from build123d import *

# Parameters (mm, degrees)
SKETCH1_W          = 201.20864
SKETCH1_H          = 290.83
BASE_FLANGE1_DEPTH = 3.175
EDGE_FLANGE1_DEPTH = 93.921520056


# Sheet-metal steps are written as plain solids
with BuildPart() as part:
    # Sketch1 → Base-Flange1 (new body)
    with BuildSketch(Plane(origin=(0, 0, 0), x_dir=(1, 0, 0), z_dir=(0, 1, 0))):
        with Locations((100.60432, 145.415)):
            Rectangle(SKETCH1_W, SKETCH1_H)
    extrude(amount=-BASE_FLANGE1_DEPTH)

    # Edge-Flange1 section (across the edge) → Edge-Flange1 (add)
    with BuildSketch(Plane(origin=(93.921520056, 0, -294.005), x_dir=(0, 0, 1), z_dir=(-1, 0, 0))):
        with BuildLine():
            Line((-3.175, 3.175), (-3.175, 34.925))
            Line((-3.175, 34.925), (0, 34.925))
            Line((0, 34.925), (0, 3.175))
            ThreePointArc((0, 3.175), (0.92993597, 0.92993597), (3.175, 0))
            Line((3.175, 0), (3.175, -3.175))
            ThreePointArc((3.175, -3.175), (-1.315128061, -1.315128061), (-3.175, 3.175))
        make_face()
    extrude(amount=EDGE_FLANGE1_DEPTH)


solid = part.part
Model file for the job. Use its own axes, mm. A direction names the side the tool comes from. Round coordinates to 2 decimals unless told otherwise and drop trailing zeros. Order: outer loops, then holes, each group sorted by start corner. A loop starts at its lowest first (then second) coordinate and runs counter-clockwise, first axis right, second up.
(1) Band-saw the part on A-A (x = 54). List the corners of the cut face in (y, z) (3 decimals).
(2) Band-saw the part on B-B (y = 24). List the corners of the cut face in (x, z) (3 decimals).
(3) Band-saw the part on C-C (z = -226). List the corners of the cut face in (x, y) (3 decimals), then the cut area to 3 significant figures.
(4) Drill centre lines: line 1 (Z direction, x = 50, y = 30) (3 decimals); line 2 (Y direction, x = 50, z = -212) (3 decimals). Where is each one in solid material? Low to high.
(5) Pin check, flat tips, straight feed: pin 1 (1.9 mm diameter, centred on y = 18.5, z = -295.5, fed in from +X); pin 2 (16 mm diameter, centred on x = 51, y = 24, fed in from +Z) (3 decimals); pin 3 (1.6 mm diameter, centred on x = 155, y = -2.5, fed in from -Z). Stop position of each tip, or through.
(6) 3-axis set-ups, long thin cutter, end or side, ignore diameter. For faces 1 (the face through (48, 19, -294.005)), 2 (the face through (93.922, 16, -295)), 3 (the face through (0, -1, -148)): which of +Z, -Z, +X, -X, +Y, -Y reach the whole face in a straight line?
Verdict:
1. outline: (-3.175, -290.83) arc R6.35 ccw to (3.175, -297.18) - (34.925, -297.18) - (34.925, -294.005) - (3.175, -294.005) arc R3.175 cw to (0, -290.83) - (0, 0) - (-3.175, 0) - close
2. outline: (0, -297.18) - (93.922, -297.18) - (93.922, -294.005) - (0, -294.005) - close
3. outline: (0, -3.175) - (201.209, -3.175) - (201.209, 0) - (0, 0) - close
3. area: 639 mm2
4. line 1: z = -297.18 to -294.005
4. line 2: y = -3.175 to 0
5. pin 1: stops at x = 93.92
5. pin 2: stops at z = -294.005
5. pin 3: stops at z = -290.83
6. face 1: +Z, +X, -X, +Y
6. face 2: -Z, +X, +Y, -Y
6. face 3: +Z, -Z, -X, +Y, -Y
